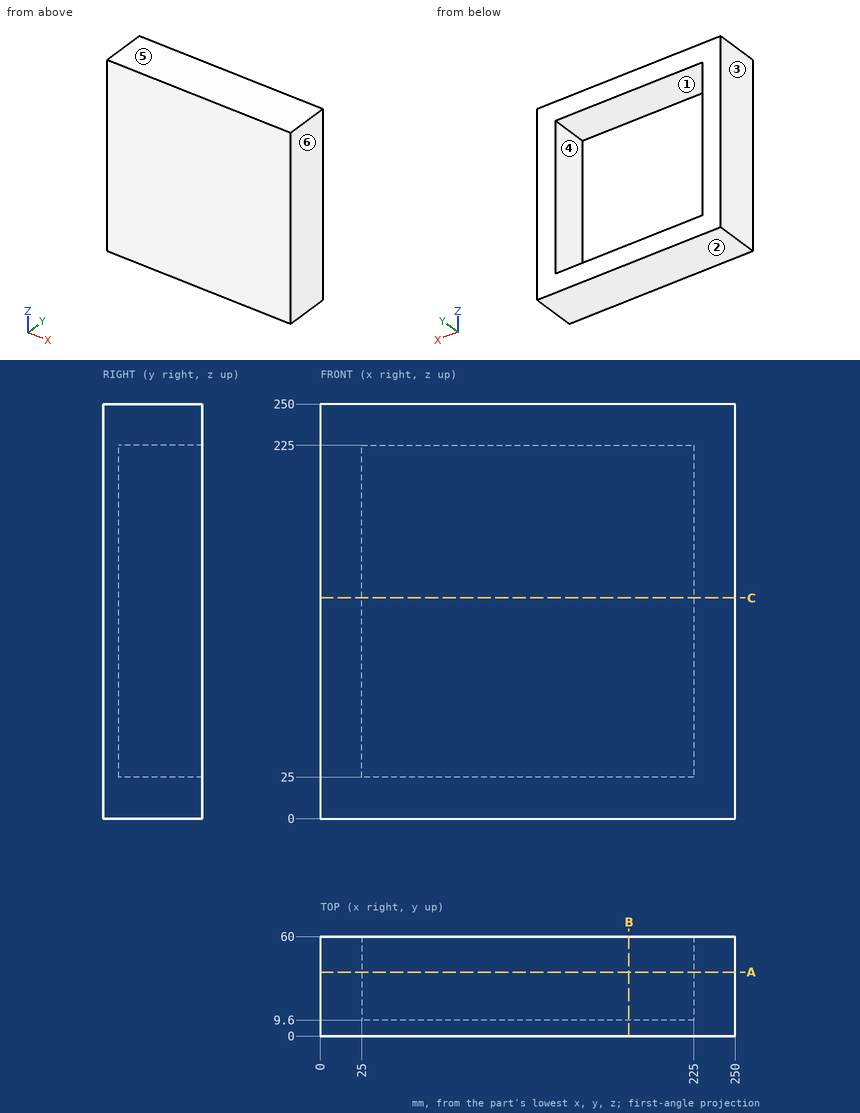
Part print with two shaded views. Sizes in mm from the minimum x, y, z corner. A direction names the side the tool comes from. Coordinates: 2 decimals unless noted, no trailing zeros. Write each loop counter-clockwise with the first axis right and the second up, starting at its lowest first coordinate (ties: lowest second). Pieces come first, ordered by that corner, then holes.
1. Drill centre lines: probe 1 along X at (y, z) = (41, 81); probe 2 along Y at (x, z) = (199.5, 67). Where is each one in solid material? Low to high.
Answer block:
probe 1: x = 0 to 25, 225 to 250
probe 2: y = 0 to 9.6
2. Band-saw the part on B-B, the plane x = 186. Give the cut face in (y, z), and give its area (3 significant figures).
Answer block:
outline: (0, 0) - (60, 0) - (60, 25) - (9.6, 25) - (9.6, 225) - (60, 225) - (60, 250) - (0, 250) - close
area: 4,920 mm2
3. Pull direction X, two halves, no side cores. Call the marked faces 3, 4, 5 and 6: released by +X, released by -X, zero draft, split by the parting line, or undercut.
Answer block:
face 3: released by -X
face 4: undercut
face 5: zero draft
face 6: released by +X
4. 3-axis set-ups, long thin cutter, end or side, ignore diameter. For the marked faces 1 and 2: which of +Z, -Z, +X, -X, +Y, -Y reach the whole face in a straight line?
Answer block:
face 1: +Y
face 2: -Z, +X, -X, +Y, -Y
5. Band-saw the part on A-A, the plane y = 38.5. Give the cut face in (x, z), and give its area (3 significant figures).
Answer block:
outline: (0, 0) - (250, 0) - (250, 250) - (0, 250) - close; hole (25, 25) - (225, 25) - (225, 225) - (25, 225) - close
area: 22,500 mm2
6. Drop flat-ended pins along their axis: pin 1 (8 mm diameter, centred on y = 35, z = 90.5, fed in from -X); pin 2 (1 mm diameter, centred on x = 197, z = 214, fed in from +Y). Give the stop position or say it passes through.
Answer block:
pin 1: stops at x = 0
pin 2: stops at y = 9.6
7. Band-saw the part on C-C, the plane z = 133. Give the cut face in (x, y), and give its area (3 significant figures).
Answer block:
outline: (0, 0) - (250, 0) - (250, 60) - (225, 60) - (225, 9.6) - (25, 9.6) - (25, 60) - (0, 60) - close
area: 4,920 mm2
